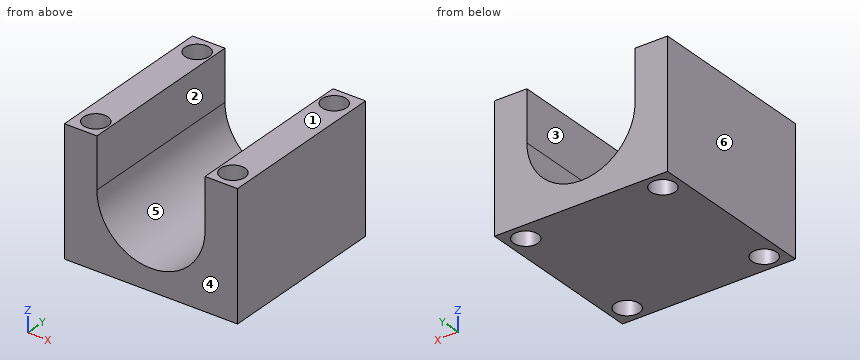
from build123d import *

# Parameters (mm, degrees)
F0_W            = 24
F0_H            = 24
F1_DEPTH        = 17.5
F3_DEPTH        = 25
F5_D            = 3.4
F5_COPIES_COUNT = 4


# Not quite as in the source:
# - a pattern or mirror of a feature is missing from the dataset's text; its kind, count and spacing are read off the source's solid


with BuildPart() as f1:
    # F0 (on Top) → F1 (new body)
    with BuildSketch(Plane.XY):
        Rectangle(F0_W, F0_H)
    extrude(amount=F1_DEPTH)

    # F2 (on face) → F3 (cut)
    with BuildSketch(Plane.XZ.offset(12)):
        with BuildLine():
            ThreePointArc((-7.5, 10.5), (0, 3), (7.5, 10.5))
            Line((7.5, 10.5), (-7.5, 10.5))
        make_face()
        with BuildLine():
            ThreePointArc((7.5, 10.5), (6.1824092402, 14.7459175671), (2.6925824036, 17.5))
            Line((2.6925824036, 17.5), (-2.6925824036, 17.5))
            ThreePointArc((-2.6925824036, 17.5), (-6.1824092402, 14.7459175671), (-7.5, 10.5))
            Line((-7.5, 10.5), (7.5, 10.5))
        make_face()
        with BuildLine():
            Line((7.5, 10.5), (7.5, 17.5))
            Line((7.5, 17.5), (2.6925824036, 17.5))
            ThreePointArc((2.6925824036, 17.5), (6.1824092402, 14.7459175671), (7.5, 10.5))
        make_face()
        with BuildLine():
            ThreePointArc((-7.5, 10.5), (-6.1824092402, 14.7459175671), (-2.6925824036, 17.5))
            Line((-2.6925824036, 17.5), (-7.5, 17.5))
            Line((-7.5, 17.5), (-7.5, 10.5))
        make_face()
    extrude(amount=-F3_DEPTH, mode=Mode.SUBTRACT)

    # F5 (through all)
    with Locations(Plane.XY.offset(17.5)):
        with Locations((-9.5, -9.5)):
            f5 = Hole(F5_D / 2)

    # F5_copies: F5 ×4 about axis
    f5_copies_axis = Axis((0, 0, 0), (0, 0, 1))
    for i in range(1, F5_COPIES_COUNT):
        add(f5.rotate(f5_copies_axis, i * 360 / F5_COPIES_COUNT), mode=Mode.SUBTRACT)


solid = f1.part
Source: CAD feature listing. Evaluate the final solid. Frame: model axes, mm. Face numbers are marked on the shaded views. A direction names the side the tool comes from. Round coordinates to 2 decimals unless told otherwise and drop trailing zeros. Loops run counter-clockwise (first coordinate to the right, second up) from the corner with the lowest first, then second, coordinate; pieces in that order, holes last.
Q1. Mould query, pull axis X, two halves, no side actions, for the marked faces 3, 4, 5 and 6. Classes: pulls with the +X half, pulls with the -X half, needs draft (parallel to the pull), parting line crosses it, or undercut.
Q2. Section B-B, the plane x = -9.5. Return loops of the section in (y, z).
Q3. Section A-A, the plane y = 9.5. Return loops of the section in (x, z).
Q4. Section C-C, the plane z = 3.5. Return loops of the section in (x, y).
Q5. Ray query, line 1 (X direction, y = 9.5, z = 11.25); line 2 (Y direction, x = 9.5, z = 7.25); line 3 (X direction, y = 9.5, z = 4.75). Return the intervals inside material, ascending.
Q6. Section D-D, the plane y = -7. Return loops of the section in (x, z), plus the area to 3 significant figures.
Q7. Access query for the marked faces 1 and 2. Directions: +Z, -Z, +X, -X, +Y, -Y. A direction counts if a zero-diameter tool reaches every point of the face in a straight line with its end or side. Return the directions, or none.
Q8. First-contact query: P1, Ø5, axis at x = 4.5, z = 14, coming from the -Y side. Flat tip, straight axial feed; report the tip coordinate or a pass-through.
Solutions:
1. face 3: undercut
1. face 4: needs draft
1. face 5: undercut
1. face 6: pulls with the -X half
2. outline: (-12, 0) - (-11.2, 0) - (-11.2, 17.5) - (-12, 17.5) - close; (-7.8, 0) - (7.8, 0) - (7.8, 17.5) - (-7.8, 17.5) - close; (11.2, 0) - (12, 0) - (12, 17.5) - (11.2, 17.5) - close
3. outline: (-12, 0) - (-11.2, 0) - (-11.2, 17.5) - (-12, 17.5) - close; (-7.8, 0) - (7.8, 0) - (7.8, 17.5) - (7.5, 17.5) - (7.5, 10.5) arc R7.5 cw to (-7.5, 10.5) - (-7.5, 17.5) - (-7.8, 17.5) - close; (11.2, 0) - (12, 0) - (12, 17.5) - (11.2, 17.5) - close
4. outline: (-12, -12) - (-2.69, -12) - (-2.69, 12) - (-12, 12) - close; (2.69, -12) - (12, -12) - (12, 12) - (2.69, 12) - close; hole circle Ø3.4 at (-9.5, -9.5); hole circle Ø3.4 at (-9.5, 9.5); hole circle Ø3.4 at (9.5, -9.5); hole circle Ø3.4 at (9.5, 9.5)
5. line 1: x = -12 to -11.2, -7.8 to -7.5, 7.5 to 7.8, 11.2 to 12
5. line 2: y = -12 to -11.2, -7.8 to 7.8, 11.2 to 12
5. line 3: x = -12 to -11.2, -7.8 to -4.82, 4.82 to 7.8, 11.2 to 12
6. outline: (-12, 0) - (12, 0) - (12, 17.5) - (7.5, 17.5) - (7.5, 10.5) arc R7.5 cw to (-7.5, 10.5) - (-7.5, 17.5) - (-12, 17.5) - close
6. area: 227 mm2
7. face 1: +Z, +X, -X, +Y, -Y
7. face 2: +Z, +Y, -Y
8. P1: passes through
